The model under review builds one solid part; all positions refer to its coordinate system, in mm. A direction names the side the tool comes from. Coordinates: 2 decimals unless noted, no trailing zeros.
from build123d import *

# Parameters (mm, degrees)
SKETCH1_R           = 50.8
BOSS_EXTRUDE1_DEPTH = 6.35
CHAMFER1_SIZE       = 1.27


with BuildPart() as part:
    # Sketch1 → Boss-Extrude1 (new body)
    with BuildSketch(Plane.XY):
        Circle(SKETCH1_R)
        with BuildLine():
            ThreePointArc((-13.847096774, 40.631261203), (-42.926, 0), (-13.847096774, -40.631261203))
            ThreePointArc((-13.847096774, -40.631261203), (-9.334096705, -38.412454682), (-11.552903226, -33.899454613))
            ThreePointArc((-11.552903226, -33.899454613), (-35.814, 0), (-11.552903226, 33.899454613))
            ThreePointArc((-11.552903226, 33.899454613), (-9.334096705, 38.412454682), (-13.847096774, 40.631261203))
        make_face(mode=Mode.SUBTRACT)
        with BuildLine():
            ThreePointArc((13.847096774, 40.631261203), (42.926, 0), (13.847096774, -40.631261203))
            ThreePointArc((13.847096774, -40.631261203), (9.334096705, -38.412454682), (11.552903226, -33.899454613))
            ThreePointArc((11.552903226, -33.899454613), (35.814, 0), (11.552903226, 33.899454613))
            ThreePointArc((11.552903226, 33.899454613), (9.334096705, 38.412454682), (13.847096774, 40.631261203))
        make_face(mode=Mode.SUBTRACT)
    extrude(amount=BOSS_EXTRUDE1_DEPTH)

    # Chamfer1
    chamfer1_edges = [part.edges().sort_by_distance(p)[0] for p in [
        (-9.334096705, -38.412454682, 6.35),
        (-35.814, 0, 6.35),
        (9.334096705, 38.412454682, 6.35),
        (35.814, 0, 6.35),
        (9.334096705, -38.412454682, 6.35),
        (42.926, 0, 6.35),
        (-50.8, 0, 6.35),
        (-9.334096705, 38.412454682, 6.35),
        (-42.926, 0, 6.35),
    ]]
    chamfer(chamfer1_edges, length=CHAMFER1_SIZE)

    # Sketch5 → CBORE for 1/2 Heavy Hex Bolt1 (revolve, cut)
    with BuildSketch(Plane(origin=(0, 0, 6.35), x_dir=(0, -1, 0), z_dir=(1, 0, 0))):
        Polygon((0, 0), (0, 6.35), (13.081, 6.35), (13.081, 3.175), (14.351, 3.175), (14.351, 0.5715), (14.9225, 0), align=None)
    revolve(axis=Axis((0, 0, 12.7), (0, 0, -1)), mode=Mode.SUBTRACT)


solid = part.part
(1) Consider section B-B (y = 0). Give the number of separate pieces and of enclosed holes in the cut face, then the cut area to 3 significant figures.
(2) Wall thickness on line 1 (Y direction, x = 0, z = 4.45); line 2 (X direction, y = 5.5, z = 0.5); line 3 (Y direction, x = -10.5, z = 1.25): over which ranges is each line inside the solid? List them lowest first.
(3) Insertion check: pin 1 Ø1 at (y, z) = (4.5, 3) entering from -X; pin 2 Ø3 at (y, z) = (31.5, 4.5) entering from +X; pin 3 Ø14.5 at (x, y) = (7, 2) entering from +Z. Each pin has a flat end and moves straight along its axis. Give the tip position at first contact, or say it passes through.
(4) Tool access review of faces 4 (the face through (42.92, 0.75, 2.5)), 5 (the face through (13, -3, 3.175)), 6 (the face through (-12, -10, 6.35)): name each direction out of +Z, -Z, +X, -X, +Y, -Y from which nothing blocks a thin tool from reaching the whole face with its end or side.
(5) The part is to be moulded in two halves that separate along X. For faces 1 (the face through (11, -11, 0)), 2 (the face through (-35.81, -0.62, 2.5)), 3 (the face through (-11.012, -49.592, 2.504)), say which applies: +X half, -X half, draft (parallel to the pull), parting line (faces both ways), or undercut.
Findings:
1. separate pieces: 4
1. enclosed holes: 0
1. area: 375 mm2
2. line 1: y = -50.8 to -14.35, 14.35 to 50.8
2. line 2: x = -50.5 to -42.57, -35.39 to -11.87, 11.87 to 35.39, 42.57 to 50.5
2. line 3: y = -49.7 to -40.06, -34.47 to -7.8, 7.8 to 34.47, 40.06 to 49.7
3. pin 1: stops at x = -50.64
3. pin 2: stops at x = 41
3. pin 3: stops at z = 5.96
4. face 4: +Z, -Z
4. face 5: +Z
4. face 6: +Z, +X, -X, +Y, -Y
5. face 1: draft
5. face 2: undercut
5. face 3: parting line
